The model under review builds one solid part; all positions refer to its coordinate system, in mm. A direction names the side the tool comes from. Round coordinates to 2 decimals unless told otherwise and drop trailing zeros. Write each loop counter-clockwise with the first axis right and the second up, starting at its lowest first coordinate (ties: lowest second). Pieces come first, ordered by that corner, then holes. Notation, with made-up numbers: (86.25, 3.5) - (99.25, 3.5) arc R16 cw to (99.25, 17.5) - close; hole circle Ø7 at (-23.75, -25.75). An arc over 180 degrees is marked (long way). Return JSON: item names as keys, results as strings.
from build123d import *

# Parameters (mm, degrees)
F1_DEPTH  = 7.25
F0_W      = 24
F0_H      = 8
F2_DEPTH  = 1.7
F4_DEPTH  = 10
F6_DEPTH  = 3.5
F7_R      = 5
F9_D      = 3.6
F10_DEPTH = 7


with BuildPart() as f1:
    # F0 (on Front) → F1 (new body)
    with BuildSketch(Plane.XZ):
        with BuildLine():
            Line((20, 12), (12, 12))
            ThreePointArc((12, 12), (8.4852813844, 3.5147186359), (2.86e-08, 0))
            Line((2.86e-08, 0), (20, 0))
            Line((20, 0), (20, 12))
        make_face()
        with BuildLine():
            Line((12, 12), (-12, 12))
            ThreePointArc((-12, 12), (-8.4852813641, 3.5147186156), (2.86e-08, 0))
            ThreePointArc((2.86e-08, 0), (8.4852813844, 3.5147186359), (12, 12))
        make_face()
        with BuildLine():
            Line((-12, 12), (-20, 12))
            Line((-20, 12), (-20, 0))
            Line((-20, 0), (2.86e-08, 0))
            ThreePointArc((2.86e-08, 0), (-8.4852813641, 3.5147186156), (-12, 12))
        make_face()
    extrude(amount=F1_DEPTH)



with BuildPart() as f1b:
    # F0 (on Front) → F1, piece 2 (new body)
    with BuildSketch(Plane.XZ):
        with BuildLine():
            ThreePointArc((12, 20), (0, 32), (-12, 20))
            Line((-12, 20), (12, 20))
        make_face()
    extrude(amount=F1_DEPTH)


with BuildPart() as f1_1:
    add(f1.part)

    add(f1b.part)  # F2 merges F1b
    # F0 (on Front) → F2 (join)
    with BuildSketch(Plane.XZ):
        with BuildLine():
            ThreePointArc((12, 20), (0, 32), (-12, 20))
            Line((-12, 20), (12, 20))
        make_face()
        with Locations((0, 16)):
            Rectangle(F0_W, F0_H)
        with BuildLine():
            Line((12, 12), (-12, 12))
            ThreePointArc((-12, 12), (-8.4852813641, 3.5147186156), (2.86e-08, 0))
            ThreePointArc((2.86e-08, 0), (8.4852813844, 3.5147186359), (12, 12))
        make_face()
    extrude(amount=-F2_DEPTH)

    # F3 (on face) → F4 (join)
    with BuildSketch(Plane(origin=(0, 1.7, 0), x_dir=(-1, 0, 0), z_dir=(0, 1, 0))):
        with BuildLine():
            ThreePointArc((-12, 12), (0, 0), (12, 12))
            Line((12, 12), (-12, 12))
        make_face()
    extrude(amount=F4_DEPTH)

    # F5 (on face) → F6 (join)
    with BuildSketch(Plane(origin=(0, 11.7, 0), x_dir=(-1, 0, 0), z_dir=(0, 1, 0))):
        with BuildLine():
            ThreePointArc((12, 20), (0, 32), (-12, 20))
            Line((-12, 20), (-12, 12))
            ThreePointArc((-12, 12), (0, 0), (12, 12))
            Line((12, 12), (12, 20))
        make_face()
    extrude(amount=F6_DEPTH)

    # F7
    f7_edges = [f1_1.edges().sort_by_distance(p)[0] for p in [
        (-20, -3.625, 12),
        (-20, -3.625, 0),
        (20, -3.625, 12),
        (20, -3.625, 0),
    ]]
    fillet(f7_edges, radius=F7_R)

    # F9 (through all)
    with Locations(Plane(origin=(0, 0, 0), x_dir=(1, 0, 0), z_dir=(0, 1, 0))):
        with Locations((15.7, -6), (-15.7, -6)):
            Hole(F9_D / 2)

    # F10 (add): a face of the model
    f10_faces = [f1_1.faces().sort_by_distance(p)[0] for p in [
        (0, 6.7, 12),
    ]]
    extrude(f10_faces, amount=F10_DEPTH)


solid = f1_1.part
(1) Clearance check with flat-ended pins moving along their axes: pin 1 Ø4 at (y, z) = (8.5, 17) entering from +X; pin 2 Ø6 at (x, y) = (0.5, -3.5) entering from +Z; pin 3 Ø6.5 at (y, z) = (9, 16) entering from -X; pin 4 Ø6 at (x, y) = (-7.5, 0.5) entering from +Z. State where each tip first meets the part, or that it passes through.
Filled in:
{"pin 1": "stops at x = 12", "pin 2": "stops at z = 32", "pin 3": "stops at x = -12", "pin 4": "stops at z = 31.12"}
(2) Add section A-A (z = 28). Write out the cut boundary in (x, y).
Filled in:
{"outline": "(-8.94, -7.25) - (8.94, -7.25) - (8.94, 1.7) - (-8.94, 1.7) - close; (-8.94, 11.7) - (8.94, 11.7) - (8.94, 15.2) - (-8.94, 15.2) - close"}
(3) Wall thickness on line 1 (X direction, y = -4, z = 6); line 2 (Y direction, x = -1.5, z = 22); line 3 (Y direction, x = -10, z = 2.5): over which ranges is each line inside the solid? List them lowest first.
Filled in:
{"line 1": "x = -20 to -17.5, -13.9 to 13.9, 17.5 to 20", "line 2": "y = -7.25 to 1.7, 11.7 to 15.2", "line 3": "y = -7.25 to 0"}
(4) Add section D-D (x = 5.5). Write out the cut boundary in (y, z), plus the area to 3 significant figures.
Filled in:
{"outline": "(-7.25, 0) - (0, 0) - (0, 1.33) - (15.2, 1.33) - (15.2, 30.67) - (11.7, 30.67) - (11.7, 19) - (1.7, 19) - (1.7, 30.67) - (-7.25, 30.67) - (-7.25, 20) - (0, 20) - (0, 12) - (-7.25, 12) - close", "area": "493 mm2"}
(5) For faces 1 (the flat face through (0, 0, 16)), 2 (the flat face through (-12, 0, 5)), 3 (the flat face through (0, 1.7, 24)), list the 3-axis set-ups (+Z, -Z, +X, -X, +Y, -Y) from which the entire face can be reached by the end or side of a thin tool; tool diameter is ignored.
Filled in:
{"face 1": "+X, -X, -Y", "face 2": "-Z, -X, +Y", "face 3": "+Z, +X, -X"}
(6) Add section C-C (z = 6). Write out the cut boundary in (x, y).
Filled in:
{"outline": "(-20, -7.25) - (-17.5, -7.25) - (-17.5, 0) - (-20, 0) - close; (-13.9, -7.25) - (13.9, -7.25) - (13.9, 0) - (10.39, 0) - (10.39, 15.2) - (-10.39, 15.2) - (-10.39, 0) - (-13.9, 0) - close; (17.5, -7.25) - (20, -7.25) - (20, 0) - (17.5, 0) - close"}
(7) Mouldability with a two-part tool opening along Z and no side actions: class faces 4 (the cylindrical face through (19, -4, 2)), 5 (the cylindrical face through (0, -3, 32)), 6 (the flat face through (0, -4, 20)) as released by +Z, released by -Z, zero draft, split by the parting line, or undercut.
Filled in:
{"face 4": "released by -Z", "face 5": "released by +Z", "face 6": "undercut"}
(8) Add section B-B (x = 15.7). Write out the cut boundary in (y, z).
Filled in:
{"outline": "(-7.25, 0.05) - (0, 0.05) - (0, 4.2) - (-7.25, 4.2) - close; (-7.25, 7.8) - (0, 7.8) - (0, 11.95) - (-7.25, 11.95) - close"}
